The listing builds one solid part. Answer for the finished solid, in the listing's coordinates (mm). A direction names the side the tool comes from. Round coordinates to 2 decimals unless told otherwise and drop trailing zeros. Write each loop counter-clockwise with the first axis right and the second up, starting at its lowest first coordinate (ties: lowest second). Pieces come first, ordered by that corner, then holes. Notation, with made-up numbers: (-36.5, 27) - (14.5, 27) arc R30 cw to (14.5, 62) - close; hole circle Ø11 at (24, 32.5). An arc over 180 degrees is marked (long way). Use a Markdown table: item, result. Add a question column.
1) A cutting plane is placed at D-D (x = 29). State how many separate pieces and enclosed holes the cut face has, then the cut area to 3 significant figures.
2) A tool of negligible diameter and unlimited length cuts with its end or side. For faces 4 (the flat face through (21, 25, 5)), 5 (the flat face through (3, 23, 2)), from which of +Z, -Z, +X, -X, +Y, -Y can it reach the whole face along a straight path? Write none if from no direction.
3) Each of these flat-tipped pins is pushed along its axis until it touches: P1, Ø6.5, axis at x = 22.5, z = 22.5, coming from the +Y side; P2, Ø6, axis at y = 30, z = 30, coming from the +X side; P3, Ø6, axis at x = 20, y = 20, coming from the -Z side; P4, Ø15, axis at x = 18.5, y = 25, coming from the +Z side. Where does it stop, or does it pass through?
4) A cutting plane is placed at C-C (z = 9). Give the vertices of the cut face in (x, y), then the cut area to 4 significant figures.
5) Find the intervals of material crossed by probe 1 along Y at (x, z) = (15, 29.5); probe 2 along Z at (x, y) = (1, 30), in increasing order. Write a range as from..to.
6) A cutting plane is placed at A-A (z = 30). Give the vertices of the cut face in (x, y), then the cut area to 3 significant figures.
7) A cutting plane is placed at B-B (x = 8). Give the vertices of the cut face in (y, z).
8) Determine the mould class of faces 1 (the flat face through (40, 7, 7)), 2 (the flat face through (25, 7, 8)), 3 (the conical face through (3.125, 32.504, 30.789)) for opening direction Y: +Y half, -Y half, draft (parallel to the pull), parting line (faces both ways), or undercut.
```python
from build123d import *

# Parameters (mm, degrees)
F0_W     = 5
F0_H     = 35
F0_H_2   = 5
F0_W_2   = 35
F0_R     = 2.5
F1_DEPTH = 5
F2_DEPTH = 40
F3_SIZE  = 5
F4_R     = 2.5
F5_DEPTH = 25
F6_R     = 2.5
F7_DEPTH = 25
F8_SIZE  = 2


with BuildPart() as f1:
    # F0 (on Top) → F1 (new body)
    with BuildSketch(Plane.XY):
        with Locations((2.5, 22.5)):
            Rectangle(F0_W, F0_H)
        with Locations((2.5, 2.5)):
            Rectangle(F0_W, F0_H_2)
        with Locations((22.5, 2.5)):
            Rectangle(F0_W_2, F0_H_2)
        with Locations((22.5, 22.5)):
            Rectangle(F0_W_2, F0_H)
        with Locations((20, 20)):
            Circle(F0_R, mode=Mode.SUBTRACT)
        with Locations((27.5, 20)):
            Circle(F0_R, mode=Mode.SUBTRACT)
        with Locations((20, 27.6)):
            Circle(F0_R, mode=Mode.SUBTRACT)
        with Locations((27.5, 27.6)):
            Circle(F0_R, mode=Mode.SUBTRACT)
        with Locations((20, 27.6)):
            Circle(F0_R)
        with Locations((27.5, 20)):
            Circle(F0_R)
    extrude(amount=F1_DEPTH)

    # F0 (on Top) → F2 (join)
    with BuildSketch(Plane.XY):
        with Locations((2.5, 22.5)):
            Rectangle(F0_W, F0_H)
        with Locations((2.5, 2.5)):
            Rectangle(F0_W, F0_H_2)
        with Locations((22.5, 2.5)):
            Rectangle(F0_W_2, F0_H_2)
    extrude(amount=F2_DEPTH)

    # F3
    f3_edges = [f1.edges().sort_by_distance(p)[0] for p in [
        (40, 40, 2.5),
        (2.5, 40, 40),
        (40, 2.5, 40),
        (0, 0, 20),
        (0, 20, 0),
        (20, 0, 0),
        (5, 22.5, 5),
        (5, 5, 22.5),
        (22.5, 5, 5),
    ]]
    chamfer(f3_edges, length=F3_SIZE)

    # F4 (on face) → F5 (cut)
    with BuildSketch(Plane.YZ.offset(5)):
        with Locations((30, 30)):
            Circle(F4_R)
        with Locations((22.5, 22.5)):
            Circle(F4_R)
    extrude(amount=-F5_DEPTH, mode=Mode.SUBTRACT)

    # F6 (on face) → F7 (cut)
    with BuildSketch(Plane(origin=(0, 5, 0), x_dir=(-1, 0, 0), z_dir=(0, 1, 0))):
        with Locations((-22.5, 22.5)):
            Circle(F6_R)
        with Locations((-30, 30)):
            Circle(F6_R)
    extrude(amount=-F7_DEPTH, mode=Mode.SUBTRACT)

    # F8
    f8_edges = [f1.edges().sort_by_distance(p)[0] for p in [
        (5, 27.5, 30),
        (5, 20, 22.5),
        (25, 5, 22.5),
        (32.5, 5, 30),
        (17.5, 20, 5),
        (25, 27.6, 5),
    ]]
    chamfer(f8_edges, length=F8_SIZE)


solid = f1.part
```
Entries:
| question | item | result |
|---|---|---|
| 1 | separate pieces | 3 |
| 1 | enclosed holes | 0 |
| 1 | area | 323 mm² |
| 2 | face 4 | +Z, +X, +Y |
| 2 | face 5 | -Z, -X, +Y, -Y |
| 3 | P1 | stops at y = 3.75 |
| 3 | P2 | stops at x = 3.5 |
| 3 | P3 | stops at z = 0 |
| 3 | P4 | stops at z = 5 |
| 4 | outline | (0, 5) - (5, 0) - (40, 0) - (40, 6) - (10, 6) - (6, 10) - (6, 40) - (0, 40) - close |
| 4 | area | 439.5 mm² |
| 5 | probe 1 | y = 0..5 |
| 5 | probe 2 | z = 4..27.5, 32.5..40 |
| 6 | outline | (0, 5) - (5, 0) - (27.5, 0) - (27.5, 3) - (25.5, 5) - (10, 5) - (5, 10) - (5, 25.5) - (3, 27.5) - (0, 27.5) - close; (0, 32.5) - (3, 32.5) - (5, 34.5) - (5, 40) - (0, 40) - close; (32.5, 0) - (40, 0) - (40, 5) - (34.5, 5) - (32.5, 3) - close |
| 6 | area | 317 mm² |
| 7 | outline | (0, 5) - (5, 0) - (40, 0) - (40, 7) - (10, 7) - (7, 10) - (7, 40) - (0, 40) - close |
| 8 | face 1 | draft |
| 8 | face 2 | +Y half |
| 8 | face 3 | undercut |
